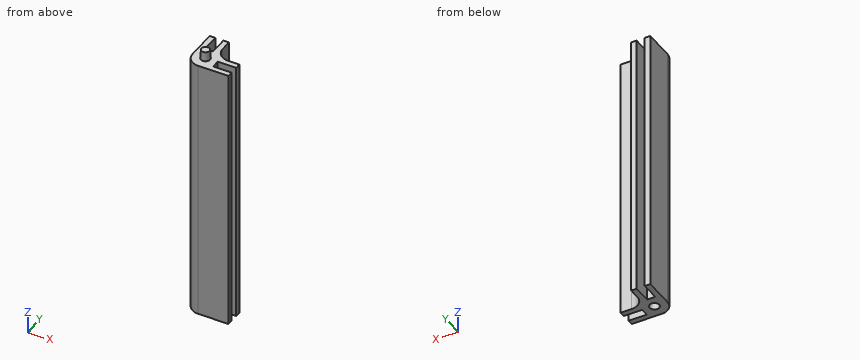
from build123d import *

# Parameters (mm, degrees)
EXTRUDE1_DEPTH     = 144.8
SKETCH2_R          = 2.5
EXTRUDE2_DEPTH     = 5
EXTRUDE2_TAPER     = 4
SKETCH3_R          = 2.6
CUT_EXTRUDE1_DEPTH = 5.2
CUT_EXTRUDE1_DRAFT = -3.8


with BuildPart() as part:
    # Sketch1 → Extrude1 (new body)
    with BuildSketch(Plane.XY):
        with BuildLine():
            Line((-3.4, -10.4), (13, -10.4))
            Line((13, -10.4), (13, -7.4))
            Line((13, -7.4), (3, -7.4))
            Line((3, -7.4), (3, -3))
            Line((3, -3), (13, -3))
            Line((13, -3), (13, 0))
            Line((13, 0), (7, 0))
            ThreePointArc((7, 0), (2.050252532, 2.050252532), (0, 7))
            Line((0, 7), (0, 13))
            Line((0, 13), (-3, 13))
            Line((-3, 13), (-3, 3))
            Line((-3, 3), (-7.4, 3))
            Line((-7.4, 3), (-7.4, 13))
            Line((-7.4, 13), (-10.4, 13))
            Line((-10.4, 13), (-10.4, -3.4))
            ThreePointArc((-10.4, -3.4), (-8.349747468, -8.349747468), (-3.4, -10.4))
        make_face()
    extrude(amount=EXTRUDE1_DEPTH)

    # Sketch2 → Extrude2 (add)
    with BuildSketch(Plane.XY.offset(144.8)):
        with Locations((-3.4, -3.4)):
            Circle(SKETCH2_R)
    extrude(amount=EXTRUDE2_DEPTH, taper=EXTRUDE2_TAPER)


with BuildPart() as cut_extrude1_tool:
    # Sketch3 → Cut-Extrude1 (with draft: the straight prism first)
    with BuildSketch(Plane(origin=(0, 0, 0), x_dir=(-1, 0, 0), z_dir=(0, 0, -1))):
        with Locations((3.4, -3.4)):
            Circle(SKETCH3_R)
    extrude(amount=-CUT_EXTRUDE1_DEPTH)
    # Cut-Extrude1: the draft: its side faces are tilted about the plane it starts from
    cut_extrude1_sides = [cut_extrude1_tool.faces().sort_by_distance(p)[0] for p in [
        (-0.8, -3.4, 2.6),
    ]]
    draft(cut_extrude1_sides, Plane(origin=(0, 0, 0), x_dir=(-1, 0, 0), z_dir=(0, 0, -1)), CUT_EXTRUDE1_DRAFT)


with BuildPart() as part_1:
    add(part.part)

    # Cut-Extrude1: cut by cut_extrude1_tool
    add(cut_extrude1_tool.part, mode=Mode.SUBTRACT)


solid = part_1.part
Work out the finished part from the listing and answer in its coordinate system (mm). Give positions to 0.01 mm unless a question says otherwise; leave off trailing zeros. Loops run counter-clockwise (first coordinate to the right, second up) from the corner with the lowest first, then second, coordinate; pieces in that order, holes last. Notation, with made-up numbers: (-27, -26) -> (25, -26) arc R29 cw to (25, 4) -> close; hole circle Ø5 at (-18, 17.5). An arc over 180 degrees is marked (long way). Use a Markdown table: item, result. Add a question column.
1) The part is cut by section B-B, the plane x = 5.75. Determine the outline of the cut face in (y, z).
2) Consider line 1 along Y through (x, z) = (11.75, 115); line 2 along Z through (x, y) = (-4.75, -0.75). Determine where each line is inside the solid, lowest interval first.
3) Each of these flat-tipped pins is pushed along its axis until it touches: P1, Ø5, axis at y = 10, z = 42, coming from the +X side; P2, Ø3.5, axis at x = -3.5, y = -3, coming from the -Z side; P3, Ø3, axis at x = 5.5, z = 76.5, coming from the +Y side. Where does it stop, or does it pass through?
4) The part is cut by section A-A, the plane z = 115. Determine the outline of the cut face in (x, y).
Reported:
| question | item | result |
|---|---|---|
| 1 | outline | (-10.4, 0) -> (-7.4, 0) -> (-7.4, 144.8) -> (-10.4, 144.8) -> close; (-3, 0) -> (0.11, 0) -> (0.11, 144.8) -> (-3, 144.8) -> close |
| 2 | line 1 | y = -10.4 to -7.4, -3 to 0 |
| 2 | line 2 | z = 0 to 144.8 |
| 3 | P1 | stops at x = 0 |
| 3 | P2 | stops at z = 5.2 |
| 3 | P3 | stops at y = 0.68 |
| 4 | outline | (-10.4, -3.4) arc R7 ccw to (-3.4, -10.4) -> (13, -10.4) -> (13, -7.4) -> (3, -7.4) -> (3, -3) -> (13, -3) -> (13, 0) -> (7, 0) arc R7 cw to (0, 7) -> (0, 13) -> (-3, 13) -> (-3, 3) -> (-7.4, 3) -> (-7.4, 13) -> (-10.4, 13) -> close |
